Work out the finished part from the listing and answer in its coordinate system (mm). A direction names the side the tool comes from. Coordinates: 2 decimals unless noted, no trailing zeros. Loops run counter-clockwise (first coordinate to the right, second up) from the corner with the lowest first, then second, coordinate; pieces in that order, holes last. Notation, with made-up numbers: M -15.75,59.5 L 23.25,59.5 A9 cw 23.25,74.5 Z; hole C 84,3 d10. An arc over 180 degrees is marked long. Write each question's results on one line, items separated by ' | '.
Autodesk Inventor part; units mm, degrees
ref_plane "YZ Plane" through (0, 0, 0) normal (1, 0, 0) x (0, 1, 0)
ref_plane "XZ Plane" through (0, 0, 0) normal (0, 1, 0) x (-1, 0, 0)
ref_plane "XY Plane" through (0, 0, 0) normal (0, 0, 1) x (1, 0, 0)
sketch "Sketch1" plane through (0, 0, 0) normal (0, 1, 0) x (-1, 0, 0)
  line L0 (-1.75, -4) -> (1.75, -4)
  line L1 (1.75, -4) -> (1.75, 4)
  line L2 (1.75, 4) -> (-1.75, 4)
  line L3 (-1.75, 4) -> (-1.75, -4)
  line L4 (-1.75, -4) -> (1.75, 4) construction
  line L5 (1.75, -4) -> (-1.75, 4) construction
  point P0 (0, 0)
  dimension "d0" = 3.5
  dimension "d1" = 8
extrude "Extrusion1" add sketch "Sketch1" along normal blind 10
sketch "Sketch2" plane through (1.75, 0, 4) normal (1, 0, 0) x (0, 0, -1)
  line L0 (2, 2.5) -> (6, 2.5)
  line L1 (6, 2.5) -> (6, 0.5)
  line L2 (6, 0.5) -> (2, 0.5)
  line L3 (2, 0.5) -> (2, 2.5)
  line L4 (8, 0) -> (8, 10)
  line L5 (0, 0) -> (8, 0)
  point P0 (4, 0)
  dimension "d4" = 2
  dimension "d5" = 4
  dimension "d6" = 2
  dimension "d7" = 0.5
extrude "Extrusion2" add sketch "Sketch2" along normal blind 5
sketch "Sketch3" plane through (1.75, 0.5, -2) normal (0, -1, 0) x (1, 0, 0)
  line L0 (5, 4) -> (5, 0)
  line L1 (0, 0) -> (5, 0)
  line L2 (5, 4) -> (3, 4)
  line L3 (3, 4) -> (3, 0)
  line L4 (3, 0) -> (5, 0)
  line L5 (5, 0) -> (5, 4)
  point P0 (-1.75, 2)
  dimension "d22" = 2
extrude "Extrusion3" add sketch "Sketch3" along normal blind 7
chamfer "Chamfer1" distance 0.8 angle 45 1 edges at (6.75, 2.5, 0)
sketch "Sketch6" plane through (4.75, 0.5, -2) normal (-1, 0, 0) x (0, 0, 1)
  line L0 (0, -7) -> (4, -7)
  line L1 (0, 0) -> (0, -7)
  line L2 (4, -7) -> (0, -7)
  line L3 (0, -7) -> (0, -5.5)
  line L4 (0, -5.5) -> (4, -5.5)
  line L5 (4, -5.5) -> (4, -7)
  point P0 (2, -0.5)
  dimension "d23" = 1.5
extrude "Extrusion6" add sketch "Sketch6" along normal blind 3
chamfer "Chamfer2" distance 1.5 angle 45 1 edges at (1.75, -6.5, 0)
properties part number "prueba_up"
1) Find section A-A, the plane x = 4.5. Give the vertices of the cut face in (y, z), and give its area (3 significant figures).
Check result:
outline: M -6.5,-2 L -5,-2 L -5,2 L -6.5,2 Z; M 0.5,-2 L 2.5,-2 L 2.5,2 L 0.5,2 Z | area: 14.0 mm^2
2) Given pin 1 Ø4.5 at (x, z) = (4.5, 1) entering from +Y; pin 2 Ø2.5 at (x, y) = (3.5, 0) entering from -Z; pin 3 Ø4.5 at (y, z) = (-2.5, -1) entering from -X, each flat-ended and moving along its own axis, determine where each tip first touches the part or whether it passes through.
Check result:
pin 1: y = 2.5 | pin 2: z = -2 | pin 3: x = 4.75
3) Find section D-D, the plane x = 2.5. Give the vertices of the cut face in (y, z).
Check result:
outline: M -5.75,-2 L -5,-2 L -5,2 L -5.75,2 Z; M 0.5,-2 L 2.5,-2 L 2.5,2 L 0.5,2 Z
4) For a pull along Y with two mould halves and no side action, classify faces 4 (the face through (5, -6.5, 0)), 5 (the face through (6.34, 2.11, 0.03)), 6 (the face through (5, -2, 2)), 7 (the face through (3, 0.5, 0)) as released by +Y, released by -Y, zero draft, split by the parting line, or undercut.
Check result:
face 4: released by -Y | face 5: released by +Y | face 6: zero draft | face 7: undercut
5) Straight lines are drawn through the part: probe 1 along X at (y, z) = (3.5, -3.5); probe 2 along Z at (x, y) = (5.5, 1.75); probe 3 along Y at (x, z) = (-0.25, -3.5). For each, find the intervals that lie inside material, in ascending order. Write a range as [from, to].
Check result:
probe 1: [-1.75, 1.75] | probe 2: [-2, 2] | probe 3: [0, 10]
6) Find section C-C, the plane y = -2. Give the vertices of the cut face in (x, z).
Check result:
outline: M 4.75,-2 L 6.75,-2 L 6.75,2 L 4.75,2 Z
7) Which of the six approach directions +Z, -Z, +X, -X, +Y, -Y give full straight-line access (tool end or side, diameter ignored) to faces 1 (the face through (3, -5, 0)), 2 (the face through (4, 2.5, 0)), 3 (the face through (5, -2, -2))?
Check result:
face 1: +Z, -Z, -X | face 2: +Z, -Z, +X, +Y | face 3: -Z, +X, +Y, -Y
